Read the model definition and answer for the solid it produces. Units are mm, in the model's axes. Coordinates: 2 decimals unless noted, no trailing zeros. Order: outer loops, then holes, each group sorted by start corner. A loop starts at its lowest first (then second) coordinate and runs counter-clockwise, first axis right, second up. Notation, with made-up numbers: M 7.5,84.5 L 34.5,84.5 A37 ccw 34.5,121.5 Z; hole C 54,64.5 d2. An arc over 180 degrees is marked long. Write each question's results on one line, items separated by ' | '.
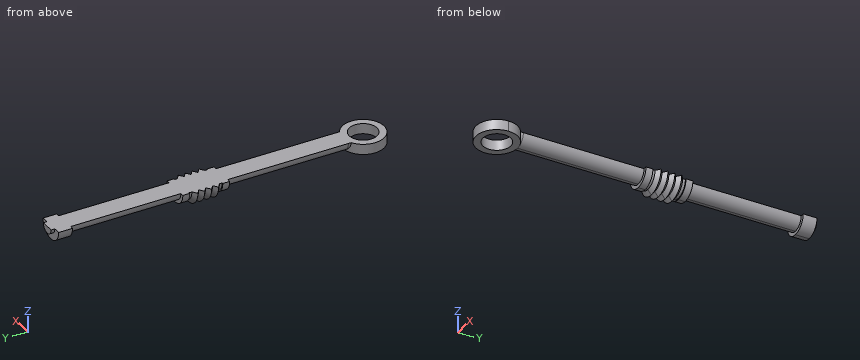
```python
from build123d import *
from build123d.topology import SkipClean

# Parameters (mm, degrees)
BOSS_EXTRUDE1_DEPTH                  = 4.7625
BOSS_EXTRUDE1_DEPTH_BACK             = 2.38125
SKETCH1_R                            = 4.7625
SKETCH1_R_2                          = 3.175
SKETCH2_R                            = 2.38125
BOSS_EXTRUDE2_DEPTH                  = 28.575
BOSS_EXTRUDE2_DIRECTION_2_REACH      = 13.666
BOSS_EXTRUDE2_DIRECTION_2_END_RADIUS = 4.7625
SKETCH3_W                            = 3.175
SKETCH3_H                            = 1.5875
BOSS_EXTRUDE3_START                  = 25.4
SKETCH4_R                            = 2.38125
BOSS_EXTRUDE3_DEPTH                  = 25.4
SKETCH5_R                            = 3.175
BOSS_EXTRUDE4_DEPTH                  = 3.175
SKETCH6_R                            = 1.5875
BOSS_EXTRUDE5_DEPTH                  = 0.83185
SKETCH7_W                            = 15.534712676
SKETCH7_H                            = 81.822586025
CUT_EXTRUDE1_DEPTH                   = 74.056725452


with BuildPart() as part:
    # Sketch1 → Boss-Extrude1 (new, two sides: drawn at the far end of the back side and taken through both)
    with BuildSketch(Plane.XY.offset(-BOSS_EXTRUDE1_DEPTH_BACK)):
        Circle(SKETCH1_R)
        Circle(SKETCH1_R_2, mode=Mode.SUBTRACT)
    extrude(amount=BOSS_EXTRUDE1_DEPTH + BOSS_EXTRUDE1_DEPTH_BACK)

    # Sketch2 → Boss-Extrude2 (add)
    with BuildSketch(Plane(origin=(0, 4.7625, 0), x_dir=(1, 0, 0), z_dir=(0, 1, 0))):
        with Locations(Location((0, 0, 0), (0, 0, 90.000000028))):
            Circle(SKETCH2_R)
    extrude(amount=BOSS_EXTRUDE2_DEPTH)

    # Boss-Extrude2 direction 2: up to this cylinder (the profile starts outside it)
    boss_extrude2_direction_2_end = Plane(origin=(0, 0, 0), z_dir=(0, 0, 1)) * Cylinder(BOSS_EXTRUDE2_DIRECTION_2_END_RADIUS, 37.857, mode=Mode.PRIVATE)
    # Sketch2 → Boss-Extrude2 direction 2 (add, up to the surface)
    with BuildSketch(Plane(origin=(0, 4.7625, 0), x_dir=(1, 0, 0), z_dir=(0, 1, 0)), mode=Mode.PRIVATE) as boss_extrude2_direction_2_sk1:
        with Locations(Location((0, 0, 0), (0, 0, 90.000000028))):
            Circle(SKETCH2_R)
    boss_extrude2_direction_2_tool1 = extrude(boss_extrude2_direction_2_sk1.sketch, amount=-BOSS_EXTRUDE2_DIRECTION_2_REACH, mode=Mode.PRIVATE) - boss_extrude2_direction_2_end
    add(boss_extrude2_direction_2_tool1.solids().sort_by_distance((0, 4.7625, 0))[0])
    add(boss_extrude2_direction_2_tool1.solids().sort_by_distance((0, 4.7625, 0))[1])

    # Sketch3 → Revolve1 (revolve)
    with SkipClean():  # the faces are left unmerged after this step: merging them gives an invalid solid
        with BuildSketch(Plane(origin=(0, 0, 0), x_dir=(0, 0, -1), z_dir=(1, 0, 0)), mode=Mode.PRIVATE) as revolve1_sk:
            with Locations((-1.5875, 33.3375)):
                Rectangle(SKETCH3_W, SKETCH3_H)
            Polygon((-2.921, 34.76625), (-2.921, 34.13125), (0, 34.13125), (0, 43.33875), (-3.175, 43.33875), (-3.175, 41.75125), (-2.921, 41.75125), (-2.921, 41.11625), (-3.96875, 40.3225), (-2.921, 39.52875), (-3.96875, 38.735), (-2.921, 37.94125), (-3.96875, 37.1475), (-2.921, 36.35375), (-3.96875, 35.56), align=None)
        revolve(revolve1_sk.sketch.rotate(Axis((0, 32.54375, 0), (0, 1, 0)), 180), axis=Axis((0, 32.54375, 0), (0, 1, 0)))

    # Sketch4 → Boss-Extrude3 (add)
    with SkipClean():  # the faces are left unmerged after this step: merging them gives an invalid solid
        with BuildSketch(Plane(origin=(0, 43.33875, 0), x_dir=(1, 0, 0), z_dir=(0, 1, 0)).offset(BOSS_EXTRUDE3_START)):
            with Locations(Location((0, 0, 0), (0, 0, 90))):
                Circle(SKETCH4_R)
        extrude(amount=-BOSS_EXTRUDE3_DEPTH)

    # Sketch5 → Boss-Extrude4 (add)
    with SkipClean():  # the faces are left unmerged after this step: merging them gives an invalid solid
        with BuildSketch(Plane(origin=(0, 68.73875, 0), x_dir=(1, 0, 0), z_dir=(0, 1, 0))):
            with Locations(Location((0, 0, 0), (0, 0, 90))):
                Circle(SKETCH5_R)
        extrude(amount=BOSS_EXTRUDE4_DEPTH)

    # Sketch6 → Boss-Extrude5 (add)
    with SkipClean():  # the faces are left unmerged after this step: merging them gives an invalid solid
        with BuildSketch(Plane(origin=(0, 71.91375, 0), x_dir=(1, 0, 0), z_dir=(0, 1, 0))):
            with Locations(Location((0, 0, 0), (0, 0, 270))):
                Circle(SKETCH6_R)
        extrude(amount=BOSS_EXTRUDE5_DEPTH)

    # Sketch7 → Cut-Extrude1 (cut, through all)
    with SkipClean():  # the faces are left unmerged after this step: merging them gives an invalid solid
        with BuildSketch(Plane.XY):
            with Locations((0.627177841, 34.425750044)):
                Rectangle(SKETCH7_W, SKETCH7_H)
        extrude(amount=CUT_EXTRUDE1_DEPTH, mode=Mode.SUBTRACT)


solid = part.part
```
(1) The part is cut by section A-A, the plane y = 16. Write down the section's boundary in (x, z), then the cut area to 3 significant figures.
Conclusion:
outline: M -2.38,0 A2.38 ccw 2.38,0 Z | area: 8.91 mm²
(2) Given pin 1 (3 mm diameter, centred on x = 3, y = 27, fed in from -Z); pin 2 (1.6 mm diameter, centred on x = 1, z = -2, fed in from -Y); pin 3 (5 mm diameter, centred on x = 0, y = 56.5, fed in from -Z); pin 4 (3 mm diameter, centred on x = 0.5, y = -1.5, fed in from -Z), each flat-ended and moving along its own axis, determine where each tip first touches the part or whether it passes through.
Conclusion:
pin 1: z = -1.85 | pin 2: y = -4.76 | pin 3: z = -2.38 | pin 4: through
(3) Straight lines are drawn through the part: line 1 (X direction, y = 0, z = -1.7) (1 decimal); line 2 (Y direction, x = 0, z = -0.5) (1 decimal); line 3 (Y direction, x = -2.5, z = -0.3). For each, find the intervals that lie inside material, in ascending order.
Conclusion:
line 1: -4.8 to -3.2, 3.2 to 4.8 | line 2: -4.8 to -3.2, 3.2 to 72.7 | line 3: -4.05 to -1.96, 1.96 to 4.05, 32.54 to 43.34, 68.74 to 71.91
